CAD build for the part. Positions are in the model's coordinates, mm. Face numbers are marked on the shaded views. A direction names the side the tool comes from. Round coordinates to 2 decimals unless told otherwise and drop trailing zeros. Order: outer loops, then holes, each group sorted by start corner. A loop starts at its lowest first (then second) coordinate and runs counter-clockwise, first axis right, second up. Notation, with made-up numbers: M 37,43 L 41,43 A25 cw 41,60 Z; hole C 81,85 d3. An arc over 180 degrees is marked long. Answer as a JSON object with one key per item and string values. Group by question number.
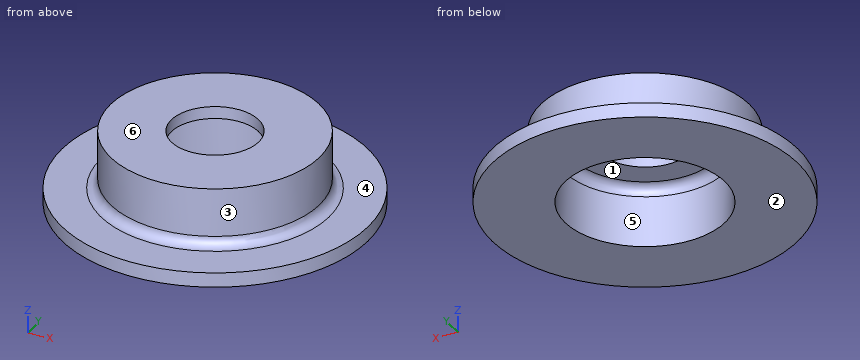
```python
from build123d import *

# Parameters (mm, degrees)
SKETCH1_R           = 12.6
BOSS_EXTRUDE1_DEPTH = 1.2
SKETCH1_3_R         = 8.6
SKETCH1_3_R_2       = 6.6
SKETCH1_3_R_3       = 3.6
BOSS_EXTRUDE2_DEPTH = 6
SKETCH1_4_R         = 6.6
SKETCH1_4_R_2       = 3.6
CUT_EXTRUDE1_DEPTH  = 5
FILLET1_R           = 0.8
FILLET2_R           = 0.8


with BuildPart() as part:
    # Sketch1 → Boss-Extrude1 (new body)
    with BuildSketch(Plane.XY):
        Circle(SKETCH1_R)
    extrude(amount=BOSS_EXTRUDE1_DEPTH)

    # Sketch1_3 → Boss-Extrude2 (add)
    # profile 1 of 2: a face of its own
    with BuildSketch(Plane.XY):
        Circle(SKETCH1_3_R)
        Circle(SKETCH1_3_R_2, mode=Mode.SUBTRACT)
    # profile 2 of 2: a face of its own
    with BuildSketch(Plane.XY):
        Circle(SKETCH1_3_R_2)
        Circle(SKETCH1_3_R_3, mode=Mode.SUBTRACT)
    extrude(amount=BOSS_EXTRUDE2_DEPTH)

    # Sketch1_4 → Cut-Extrude1 (cut)
    with BuildSketch(Plane.XY):
        Circle(SKETCH1_4_R)
        Circle(SKETCH1_4_R_2, mode=Mode.SUBTRACT)
    extrude(amount=CUT_EXTRUDE1_DEPTH, mode=Mode.SUBTRACT)


with BuildPart() as cut_extrude1_kept_piece:
    # of the separate pieces the step leaves, the one the design keeps (cut_extrude1_pieces_kept)
    add(part.part.solids().sort_by_distance((12.6, 0, 0))[0])

    # Fillet1
    fillet1_edges = [cut_extrude1_kept_piece.edges().sort_by_distance(p)[0] for p in [
        (-6.6, 0, 5),
    ]]
    fillet(fillet1_edges, radius=FILLET1_R)

    # Fillet2
    fillet2_edges = [cut_extrude1_kept_piece.edges().sort_by_distance(p)[0] for p in [
        (-8.6, 0, 1.2),
    ]]
    fillet(fillet2_edges, radius=FILLET2_R)


solid = cut_extrude1_kept_piece.part
```
Item 1: 3-axis set-ups, long thin cutter, end or side, ignore diameter. For the marked faces 4, 5 and 6: which of +Z, -Z, +X, -X, +Y, -Y reach the whole face in a straight line?
Item 2: Cut at A-A, the plane x = 0. Give the cut face in (y, z), and give its area (3 significant figures).
Item 3: Cut at C-C, the plane z = 3.75. Give the cut face in (x, y), and give its area (3 significant figures).
Item 4: Drill centre lines: line 1 (Y direction, x = 0, z = 5.15); line 2 (Y direction, x = 0, z = 3.2); line 3 (Z direction, x = -2, y = 10.75). Where is each one in solid material? Low to high. Write a range as [from, to].
Item 5: Flat gauge pins, fed straight in: pin 1 Ø2 at (x, z) = (-0.5, 5) entering from -Y; pin 2 Ø1 at (x, z) = (4.5, 4) entering from -Y; pin 3 Ø3.5 at (x, y) = (1, -2.5) entering from -Z. Where does each tip first touch, or does it go through?
Item 6: Two-plate mould, pull along Y, no slides. Class the marked faces 1, 2 and 3: +Y half, -Y half, draft (parallel to the pull), parting line (faces both ways), or undercut.
Item 7: Cut at D-D, the plane x = 9.75. Give the cut face in (y, z), and give its area (3 significant figures).
Response values:
{
 "1": {"face 4": "+Z", "face 5": "-Z", "face 6": "+Z, +X, -X, +Y, -Y"},
 "2": {"outline": "M -12.6,0 L -6.6,0 L -6.6,4.2 A0.8 cw -5.8,5 L -3.6,5 L -3.6,6 L -8.6,6 L -8.6,2 A0.8 cw -9.4,1.2 L -12.6,1.2 Z; M 3.6,5 L 5.8,5 A0.8 cw 6.6,4.2 L 6.6,0 L 12.6,0 L 12.6,1.2 L 9.4,1.2 A0.8 cw 8.6,2 L 8.6,6 L 3.6,6 Z", "area": "40.1 mm^2"},
 "3": {"outline": "C 0,0 d17.2; hole C 0,0 d13.2", "area": "95.5 mm^2"},
 "4": {"line 1": "[-8.6, -3.6], [3.6, 8.6]", "line 2": "[-8.6, -6.6], [6.6, 8.6]", "line 3": "[0, 1.2]"},
 "5": {"pin 1": "y = -8.6", "pin 2": "y = -7.61", "pin 3": "z = 5"},
 "6": {"face 1": "undercut", "face 2": "draft", "face 3": "parting line"},
 "7": {"outline": "M -7.98,0 L 7.98,0 L 7.98,1.2 L -7.98,1.2 Z", "area": "19.2 mm^2"}
}
